Here's the drawing with two shaded views (mm, measured from the low corner). I have some questions. A direction names the side the tool comes from. Give positions to 0.01 mm unless a question says otherwise; leave off trailing zeros. Write each loop counter-clockwise with the first axis right and the second up, starting at its lowest first coordinate (ties: lowest second). Pieces come first, ordered by that corner, then holes. Notation, with made-up numbers: (4, -12.5) - (13, -12.5) arc R18 cw to (13, 5.5) - close; hole circle Ø8 at (-18.5, 62.25). An arc over 180 degrees is marked (long way). Use one line per item in the form item = value.
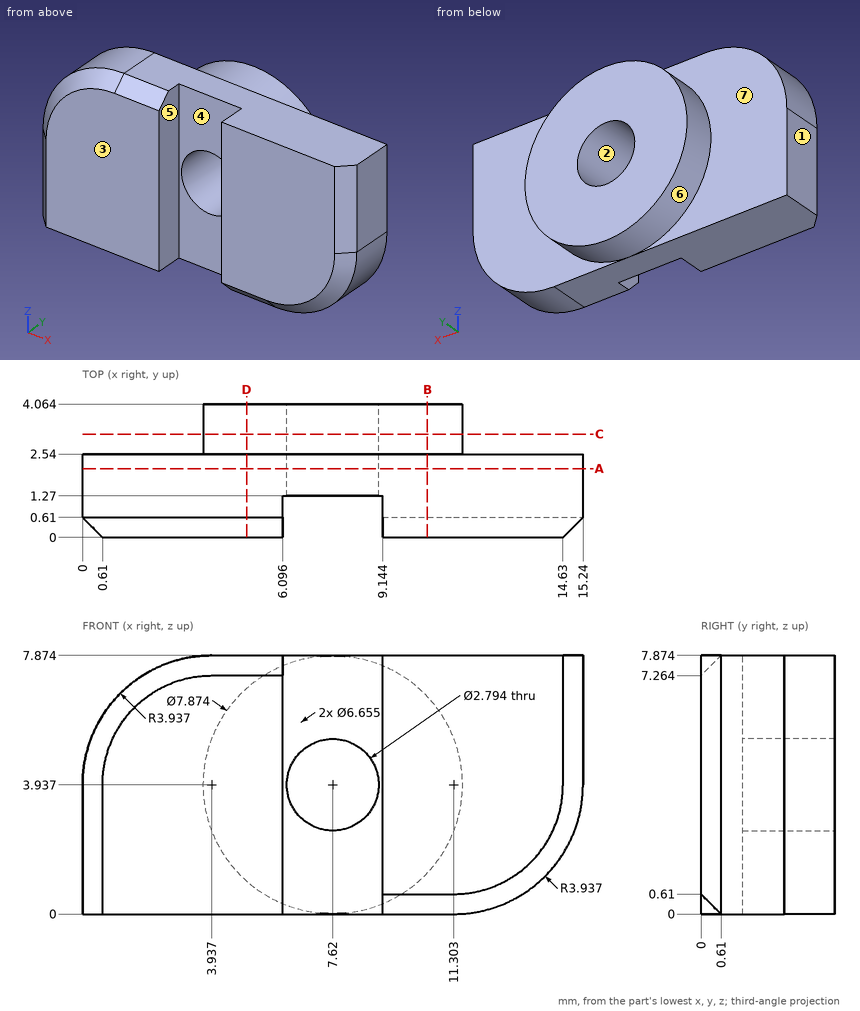
1. Imagine slicing it at A-A, the plane y = 2.1. List the corners of the cut face in (x, z) for me, and give its area (3 significant figures).
Response values:
outline = (0, 0) - (11.3, 0) arc R3.94 ccw to (15.24, 3.94) - (15.24, 7.87) - (3.94, 7.87) arc R3.94 ccw to (0, 3.94) - close; hole circle Ø2.79 at (7.62, 3.94)
area = 107 mm²
2. Imagine slicing it at B-B, the plane x = 10.5. List the corners of the cut face in (y, z) for me.
Response values:
outline = (0, 0.61) - (0.61, 0) - (2.54, 0) - (2.54, 1.25) - (4.06, 1.25) - (4.06, 6.62) - (2.54, 6.62) - (2.54, 7.87) - (0, 7.87) - close
3. Imagine slicing it at D-D, the plane x = 5. List the corners of the cut face in (y, z) for me (1 decimal).
Response values:
outline = (0, 0) - (2.5, 0) - (2.5, 1) - (4.1, 1) - (4.1, 6.9) - (2.5, 6.9) - (2.5, 7.9) - (0.6, 7.9) - (0, 7.3) - close
4. If I drill on line 1 (X direction, y = 0.3, z = 7) (1 decimal); line 2 (Y direction, x = 2.25, z = 0.75); line 3 (X direction, y = 0.2, z = 2.75) (1 decimal), over which ranges is the centre line in solid material (lowest first)? Write a range as from..to.
Response values:
line_1 = 2..6.1, 9.1..14.9
line_2 = 0..2.54
line_3 = 0.4..6.1, 9.1..14.6
5. If we mould it in two halves opening along X, with no side actions, what happens to the marked faces 1, 2, 3 and 4? For each: pulls with the +X half, pulls with the -X half, needs draft (parallel to the pull), parting line crosses it, or undercut.
Response values:
face_1 = pulls with the -X half
face_2 = undercut
face_3 = needs draft
face_4 = undercut
6. Imagine slicing it at C-C, the plane y = 3.15. List the corners of the cut face in (x, z) for me.
Response values:
outline = circle Ø7.87 at (7.62, 3.94); hole circle Ø2.79 at (7.62, 3.94)
7. Which directions (+Z, -Z, +X, -X, +Y, -Y) give clear straight access to the entire face, cutting with the end or side of a thin tool? Please do the marked faces 5, 6 and 7.
Response values:
face_5 = +Z, -Z, -Y
face_6 = +Y
face_7 = -X, +Y
8. For pin 1 (4.5 mm diameter, centred on x = 7.62, z = 3.937, fed in from +Y); pin 2 (1 mm diameter, centred on y = 1.5, z = 1.5, fed in from +X); pin 3 (1.5 mm diameter, centred on y = 1.5, z = 1, fed in from +X), each with a flat end and sliding along its axis, tell me the tip position at first contact or that it passes through.
Response values:
pin_1 = 4.06
pin_2 = 14.73
pin_3 = 14.58
